Verification items for this drawing (mm, ordinates from the low corner). A direction names the side the tool comes from. Give positions to 0.01 mm unless a question says otherwise; leave off trailing zeros. Write each loop counter-clockwise with the first axis right and the second up, starting at its lowest first coordinate (ties: lowest second). Pieces come first, ordered by that corner, then holes. Notation, with made-up numbers: M -37.75,-30 L -20.75,-30 A32 cw -20.75,-3 Z; hole C -15,42.5 d7. An arc over 180 degrees is marked long. Write each question's results on one line, items separated by ' | '.
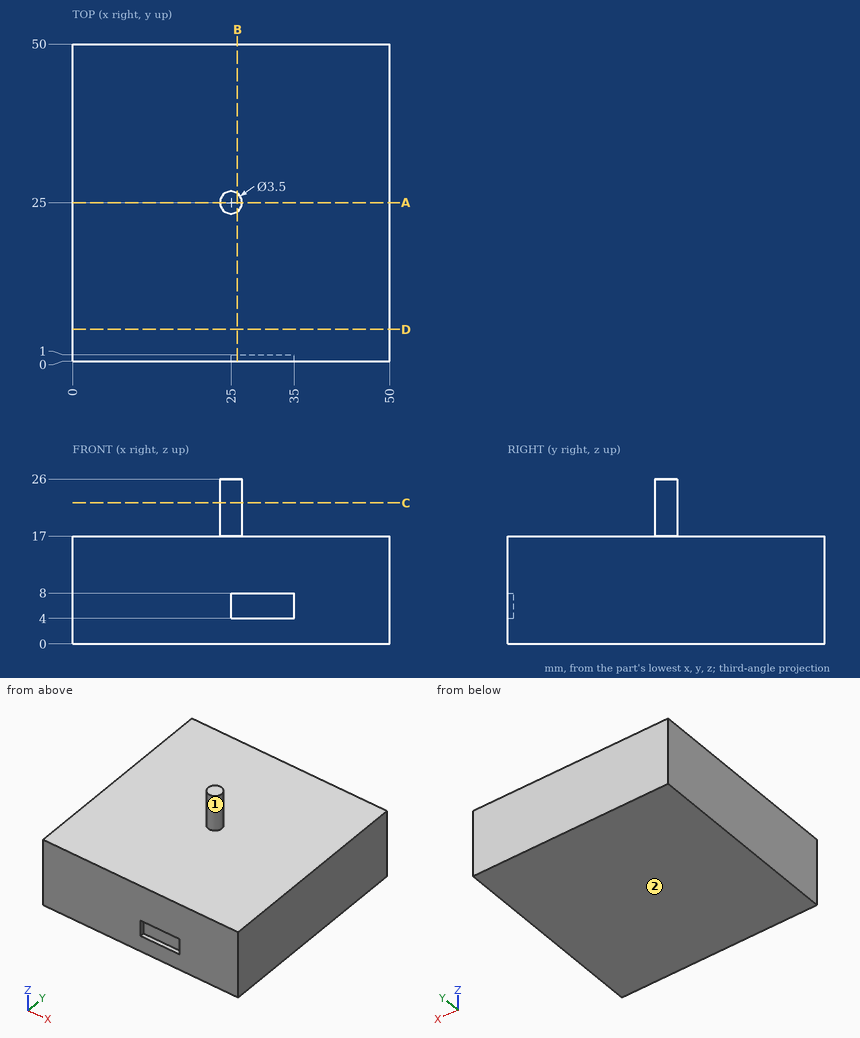
Q1. Section check A-A (y = 25). Enter the section's corners in (x, z).
Answer key:
outline: M 0,0 L 50,0 L 50,17 L 26.75,17 L 26.75,26 L 23.25,26 L 23.25,17 L 0,17 Z
Q2. Section check C-C (z = 22.25). Enter the section's corners in (x, y), then the cut area to 3 significant figures.
Answer key:
outline: C 25,25 d3.5 | area: 9.62 mm2
Q3. Section check D-D (y = 5). Enter the section's corners in (x, z).
Answer key:
outline: M 0,0 L 50,0 L 50,17 L 0,17 Z
Q4. Material ranges on probe 1 along Z at (x, y) = (10.5, 12); probe 2 along Y at (x, z) = (33, 5), recorded low to high. Write a range as [from, to].
Answer key:
probe 1: z = [0, 17] | probe 2: y = [1, 50]
Q5. Depth check by flat-ended pin: P1, Ø1, axis at x = 15, y = 15, coming from the -Z side; P2, Ø0.5, axis at x = 31.5, y = 0.5, coming from the +Z side. Enter the tip coordinate at first touch or a pass-through.
Answer key:
P1: stops at z = 0 | P2: stops at z = 17
Q6. Section check B-B (x = 26). Enter the section's corners in (y, z).
Answer key:
outline: M 0,0 L 50,0 L 50,17 L 26.44,17 L 26.44,26 L 23.56,26 L 23.56,17 L 0,17 L 0,8 L 1,8 L 1,4 L 0,4 Z
Q7. Access from +Z, -Z, +X, -X, +Y, -Y to the whole of each face (thin tool, end or side, straight path). Record for the marked faces 1 and 2.
Answer key:
face 1: +Z | face 2: -Z, +X, -X, +Y, -Y
